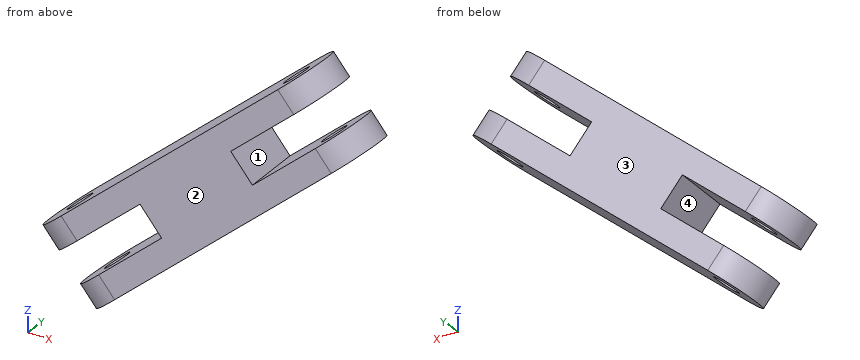
```python
from build123d import *

# Parameters (mm, degrees)
SKETCH1_R                = 1.651
BOSS_EXTRUDE1_DEPTH      = 5.334
BOSS_EXTRUDE1_DEPTH_BACK = 5.334
CUT_EXTRUDE1_DEPTH       = 10.414


with BuildPart() as part:
    # Sketch1 → Boss-Extrude1 (new body, two sides)
    with BuildSketch(Plane(origin=(10.702221059, 0, -12.754410396), x_dir=(0.766044443, 0, 0.64278761), z_dir=(-0.64278761, 0, 0.766044443))) as boss_extrude1_sk:
        with BuildLine():
            Line((-32.691973638, 7.79265549), (-1.277889133, 13.436683202))
            ThreePointArc((-1.277889133, 13.436683202), (4.178001254, 9.642679764), (0.383997817, 4.186789377))
            Line((0.383997817, 4.186789377), (-31.030086688, -1.457238335))
            ThreePointArc((-31.030086688, -1.457238335), (-36.485977075, 2.336765102), (-32.691973638, 7.79265549))
        make_face()
        with Locations((-31.861030163, 3.167708577)):
            Circle(SKETCH1_R, mode=Mode.SUBTRACT)
        with Locations((-0.446945658, 8.811736289)):
            Circle(SKETCH1_R, mode=Mode.SUBTRACT)
    extrude(amount=BOSS_EXTRUDE1_DEPTH)
    extrude(boss_extrude1_sk.sketch, amount=-BOSS_EXTRUDE1_DEPTH_BACK)

    # Sketch3 → Cut-Extrude1 (cut)
    with BuildSketch(Plane(origin=(-1.822096994, 13.238927242, -1.528920916), x_dir=(0.990782435, 0.134568376, -0.015540867), z_dir=(-0.135462786, 0.984240671, -0.113666774))):
        Polygon((-17.612221816, 34.057028648), (-6.98123986, 24.993744329), (-4.17986107, 28.279684206), (-14.810843026, 37.342968525), align=None)
        Polygon((16.629373849, 10.539082885), (5.998391893, 19.602367204), (3.197013104, 16.316427327), (13.82799506, 7.253143007), align=None)
    extrude(amount=-CUT_EXTRUDE1_DEPTH, mode=Mode.SUBTRACT)


solid = part.part
```
The model under review builds one solid part; all positions refer to its coordinate system, in mm. Face numbers are marked on the shaded views. Round coordinates to 2 decimals unless told otherwise and drop trailing zeros. Loops run counter-clockwise (first coordinate to the right, second up) from the corner with the lowest first, then second, coordinate; pieces in that order, holes last.
Item 1: Take a section at B-B (x = -6.5). Write out the cut boundary in (y, z), then the cut area to 3 significant figures.
Determined:
outline: (-0.72, -34.15) - (8.83, -34.15) - (9.31, -30.01) - (-0.24, -30.01) - close; (0.18, -26.33) - (9.43, -28.92) - (10.44, -20.23) - (0.89, -20.23) - close
area: 110 mm2
Item 2: Clearance check with flat-ended pins moving along their axes: pin 1 Ø1 at (y, z) = (7, -30.5) entering from +X; pin 2 Ø4 at (y, z) = (6, -11.5) entering from +X; pin 3 Ø8 at (x, z) = (0.5, -16) entering from -Y. State where each tip first meets the part, or that it passes through.
Determined:
pin 1: stops at x = -1.55
pin 2: stops at x = 16.18
pin 3: stops at y = 1.62
Item 3: Take a section at D-D (y = 1). Write out the cut boundary in (x, z) (3 decimals), then the cut area to 3 significant figures.
Determined:
outline: (-20.327, -31.828) - (-18.286, -34.26) - (-7.578, -25.275) - (-4.803, -28.583) - (-15.511, -37.568) - (-13.47, -40) - (0.837, -27.995) - (-6.02, -19.823) - close
area: 139 mm2
Item 4: Take a section at A-A (y = 12.5). Write out the cut boundary in (x, z), then the cut area to 3 significant figures.
Determined:
outline: (2.3, -12.84) - (4.34, -15.27) - (11.2, -9.52) - (9.16, -7.08) - close; (7.12, -18.58) - (9.16, -21.01) - (16.02, -15.26) - (13.98, -12.82) - close
area: 56.9 mm2
Item 5: For line 1 (X direction, y = 4, z = -30.5); line 2 (X direction, y = 12, z = -14); line 3 (Z direction, x = -10, y = 0.5), list the stretches that pass through material, from the lowest coordinate up.
Determined:
line 1: x = -18.74 to -17.86, -14.14 to -13.8, -7.09 to -2.15
line 2: x = 0.92 to 5.86, 12.58 to 15.67
line 3: z = -37.09 to -32.94, -27.31 to -23.16
Item 6: Mouldability with a two-part tool opening along X and no side actions: class the marked faces 1, 2, 3 and 4 as released by +X, released by -X, zero draft, split by the parting line, or undercut.
Determined:
face 1: undercut
face 2: released by +X
face 3: released by -X
face 4: undercut
Item 7: Take a section at C-C (x = 2). Write out the cut boundary in (y, z).
Determined:
outline: (1.27, -27.02) - (10.82, -27.02) - (11.8, -18.57) - (7.04, -17.24) - (11.95, -17.24) - (12.43, -13.09) - (2.88, -13.09) - close
